Could you check a few things on this model? Use its own coordinates, in mm. Face numbers are marked on the shaded views. A direction names the side the tool comes from. Give positions to 0.01 mm unless a question says otherwise; leave off trailing zeros. Loops run counter-clockwise (first coordinate to the right, second up) from the corner with the lowest first, then second, coordinate; pieces in that order, holes last. Notation, with made-up numbers: (41, 62.25) - (80, 62.25) arc R28 cw to (80, 97.25) - close; hole circle Ø10 at (65.5, 3.5). An arc over 180 degrees is marked (long way). Answer in a Markdown table with one row per item. Add a question column.
```python
from build123d import *

# Parameters (mm, degrees)
F2_R      = 32.75
F3_DEPTH  = 40
F4_R      = 30
F5_DEPTH  = 35
F7_R      = 14.5
F8_DEPTH  = 25
F9_R      = 13.305561
F10_DEPTH = 140


with BuildPart() as f1:
    # F0 (on Front) → F1 (revolve)
    with BuildSketch(Plane.XZ):
        Polygon((16.2, 140.915044), (0, 140.915044), (0, 55.007186), (34.3, 55.007186), align=None)
    revolve(axis=Axis((0, 0, 55.007186), (0, 0, 1)))

    # F2 (on face) → F3 (join)
    with BuildSketch(Plane(origin=(0, 0, 55.007186), x_dir=(1, 0, 0), z_dir=(0, 0, -1))):
        Circle(F2_R)
    extrude(amount=F3_DEPTH)

    # F4 (on face) → F5 (cut)
    with BuildSketch(Plane(origin=(0, 0, 15.007186), x_dir=(1, 0, 0), z_dir=(0, 0, -1))):
        Circle(F4_R)
    extrude(amount=-F5_DEPTH, mode=Mode.SUBTRACT)

    # F7 (on face) → F8 (join)
    with BuildSketch(Plane.XY.offset(140.915044)):
        Circle(F7_R)
    extrude(amount=F8_DEPTH)

    # F9 (on face) → F10 (cut)
    with BuildSketch(Plane.XY.offset(165.915044)):
        Circle(F9_R)
    extrude(amount=-F10_DEPTH, mode=Mode.SUBTRACT)


solid = f1.part
```
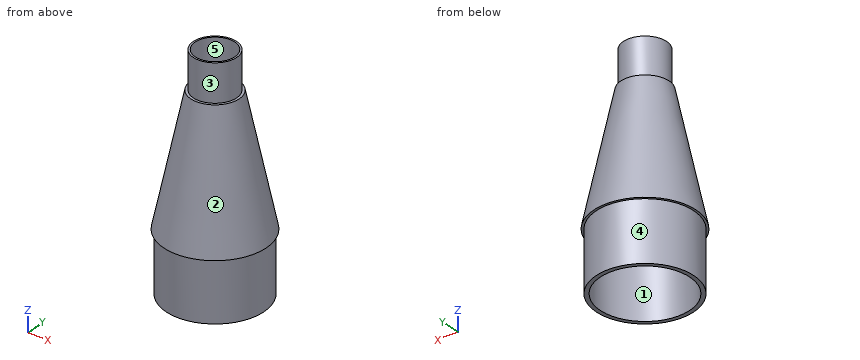
(1) I want a section at D-D on z = 149. Please give me the cut outline in (x, y).
(2) Please list where these lines run through material, in increasing order: line 1 (X direction, y = 0, z = 27); line 2 (Y direction, x = 0, z = 142).
(3) For pin 1 Ø3 at (y, z) = (15.5, 130.5) entering from -X; pin 2 Ø3 at (y, z) = (-18.5, 68.5) entering from +X; pin 3 Ø12 at (y, z) = (26, 113.5) entering from -X, each with a flat end and sliding along its axis, tell me the tip position at first contact or that it passes through.
(4) I want a section at C-C on z = 40. Please give me the cut outline in (x, y), then the cut area to 3 significant figures.
(5) We'd pull the mould along Y, two halves only. Please class the marked faces 1 and 2: pulls with the +Y half, pulls with the -Y half, needs draft (parallel to the pull), parting line crosses it, or undercut.
(6) I want a section at A-A on y = 0. Please give me the cut outline in (x, z).
(7) On a 3-axis mill with a long thin cutter (end or side, diameter ignored), from which of +Z, -Z, +X, -X, +Y, -Y can I reach the whole of each face in a straight line? I mean the marked faces 3, 4 and 5. Say none if no direction works.
Reported:
| question | item | result |
|---|---|---|
| 1 | outline | circle Ø29 at (0, 0); hole circle Ø26.61 at (0, 0) |
| 2 | line 1 | -32.75 to -30, 30 to 32.75 |
| 2 | line 2 | -14.5 to -13.31, 13.31 to 14.5 |
| 3 | pin 1 | x = -12 |
| 3 | pin 2 | x = 26.54 |
| 3 | pin 3 | x = -9.45 |
| 4 | outline | circle Ø65.5 at (0, 0); hole circle Ø60 at (0, 0) |
| 4 | area | 542 mm² |
| 5 | face 1 | undercut |
| 5 | face 2 | parting line crosses it |
| 6 | outline | (-34.3, 55.01) - (-32.75, 55.01) - (-32.75, 15.01) - (-30, 15.01) - (-30, 50.01) - (-13.31, 50.01) - (-13.31, 165.92) - (-14.5, 165.92) - (-14.5, 140.92) - (-16.2, 140.92) - close; (13.31, 50.01) - (30, 50.01) - (30, 15.01) - (32.75, 15.01) - (32.75, 55.01) - (34.3, 55.01) - (16.2, 140.92) - (14.5, 140.92) - (14.5, 165.92) - (13.31, 165.92) - close |
| 7 | face 3 | +Z |
| 7 | face 4 | -Z |
| 7 | face 5 | +Z, -Z |
